Can you work these out from the model? Positions are in its coordinate system, mm. A direction names the side the tool comes from. Round coordinates to 2 decimals unless told otherwise and drop trailing zeros. Order: outer loops, then holes, each group sorted by start corner. A loop starts at its lowest first (then second) coordinate and runs counter-clockwise, first axis right, second up. Notation, with made-up numbers: M 53.5,88.25 L 111.5,88.25 A28 ccw 111.5,116.25 Z; hole C 21,69.5 d11. An arc over 180 degrees is marked long. One line per question, with ' | ' between items.
```python
from build123d import *

# Parameters (mm, degrees)
SKETCH1_W           = 38
SKETCH1_H           = 38
BOSS_EXTRUDE1_DEPTH = 1.6
SKETCH2_W           = 17
SKETCH2_H           = 17
BOSS_EXTRUDE2_DEPTH = 3.5
SKETCH3_R           = 7.5
BOSS_EXTRUDE3_DEPTH = 12.5
CUT_EXTRUDE1_REACH  = 3.6
SKETCH4_R           = 1
SKETCH5_W           = 10
SKETCH5_H           = 5
BOSS_EXTRUDE4_DEPTH = 8


with BuildPart() as part:
    # Sketch1 → Boss-Extrude1 (new body)
    with BuildSketch(Plane.XY):
        Rectangle(SKETCH1_W, SKETCH1_H)
    extrude(amount=-BOSS_EXTRUDE1_DEPTH)

    # Sketch2 → Boss-Extrude2 (add)
    with BuildSketch(Plane.XY):
        Rectangle(SKETCH2_W, SKETCH2_H)
    extrude(amount=BOSS_EXTRUDE2_DEPTH)

    # Sketch3 → Boss-Extrude3 (add)
    with BuildSketch(Plane.XY.offset(3.5)):
        Circle(SKETCH3_R)
    extrude(amount=BOSS_EXTRUDE3_DEPTH)

    # Sketch4 → Cut-Extrude1 (cut, up to next)
    with BuildSketch(Plane.XY, mode=Mode.PRIVATE) as cut_extrude1_sk1:
        with Locations((-17, 17)):
            Circle(SKETCH4_R)
    cut_extrude1_tool1 = extrude(cut_extrude1_sk1.sketch, amount=-CUT_EXTRUDE1_REACH, mode=Mode.PRIVATE) & part.part
    add(cut_extrude1_tool1.solids().sort_by_distance((-17, 17, 0))[0], mode=Mode.SUBTRACT)
    # Sketch4 → Cut-Extrude1 (cut, up to next)
    with BuildSketch(Plane.XY, mode=Mode.PRIVATE) as cut_extrude1_sk2:
        with Locations((17, 17)):
            Circle(SKETCH4_R)
    cut_extrude1_tool2 = extrude(cut_extrude1_sk2.sketch, amount=-CUT_EXTRUDE1_REACH, mode=Mode.PRIVATE) & part.part
    add(cut_extrude1_tool2.solids().sort_by_distance((17, 17, 0))[0], mode=Mode.SUBTRACT)
    # Sketch4 → Cut-Extrude1 (cut, up to next)
    with BuildSketch(Plane.XY, mode=Mode.PRIVATE) as cut_extrude1_sk3:
        with Locations((-17, -17)):
            Circle(SKETCH4_R)
    cut_extrude1_tool3 = extrude(cut_extrude1_sk3.sketch, amount=-CUT_EXTRUDE1_REACH, mode=Mode.PRIVATE) & part.part
    add(cut_extrude1_tool3.solids().sort_by_distance((-17, -17, 0))[0], mode=Mode.SUBTRACT)
    # Sketch4 → Cut-Extrude1 (cut, up to next)
    with BuildSketch(Plane.XY, mode=Mode.PRIVATE) as cut_extrude1_sk4:
        with Locations((17, -17)):
            Circle(SKETCH4_R)
    cut_extrude1_tool4 = extrude(cut_extrude1_sk4.sketch, amount=-CUT_EXTRUDE1_REACH, mode=Mode.PRIVATE) & part.part
    add(cut_extrude1_tool4.solids().sort_by_distance((17, -17, 0))[0], mode=Mode.SUBTRACT)

    # Sketch5 → Boss-Extrude4 (add)
    with BuildSketch(Plane(origin=(0, 0, -1.6), x_dir=(-1, 0, 0), z_dir=(0, 0, -1))):
        with Locations((-5, -13.5)):
            Rectangle(SKETCH5_W, SKETCH5_H)
    extrude(amount=BOSS_EXTRUDE4_DEPTH)


solid = part.part
```
(1) If we section it at D-D on z = 0.5: Please give me the cut outline in (x, y), plus the area to 3 significant figures.
Final values:
outline: M -8.5,-8.5 L 8.5,-8.5 L 8.5,8.5 L -8.5,8.5 Z | area: 289 mm^2
(2) Will these pins go through, and if not, where does the flat tip stop? pin 1 Ø1 at (y, z) = (-0.5, 2.5) entering from +X; pin 2 Ø3 at (x, y) = (17, -17) entering from +Z; pin 3 Ø2.5 at (y, z) = (-14.5, -4.5) entering from -X.
Final values:
pin 1: x = 8.5 | pin 2: z = 0 | pin 3: x = 0
(3) If we section it at C-C on y = 0: Please give me the cut outline in (x, z).
Final values:
outline: M -19,-1.6 L 19,-1.6 L 19,0 L 8.5,0 L 8.5,3.5 L 7.5,3.5 L 7.5,16 L -7.5,16 L -7.5,3.5 L -8.5,3.5 L -8.5,0 L -19,0 Z
(4) Thinking about a two-plate mould opening in X: for faces 1 (the flat face through (5, -11, -6)), 2 (the cylindrical face through (17, -18, -1)), 3 (the cylindrical face through (-7.493, 0.33, 9.662)), which applies, released by +X, released by -X, zero draft, split by the parting line, or undercut?
Final values:
face 1: zero draft | face 2: undercut | face 3: split by the parting line
(5) Please list where these lines run through material, in increasing order: probe 1 along Y at (x, z) = (-17, -0.85); probe 2 along Z at (x, y) = (-6, 12); probe 3 along Y at (x, z) = (2, 1). Write a range as [from, to].
Final values:
probe 1: [-19, -18], [-16, 16], [18, 19] | probe 2: [-1.6, 0] | probe 3: [-8.5, 8.5]
(6) On a 3-axis mill with a long thin cutter (end or side, diameter ignored), from which of +Z, -Z, +X, -X, +Y, -Y can I reach the whole of each face in a straight line? I mean faces 4 (the flat face through (5, -16, -6)), 5 (the flat face through (0, 8.5, 2)), 6 (the flat face through (8.5, 0, 2)). Say none if no direction works.
Final values:
face 4: -Z, +X, -X, -Y | face 5: +Z, +X, -X, +Y | face 6: +Z, +X, +Y, -Y
(7) If we section it at A-A on x = -17: Please give me the cut outline in (y, z), plus the area to 3 significant figures.
Final values:
outline: M -19,-1.6 L -18,-1.6 L -18,0 L -19,0 Z; M -16,-1.6 L 16,-1.6 L 16,0 L -16,0 Z; M 18,-1.6 L 19,-1.6 L 19,0 L 18,0 Z | area: 54.4 mm^2
